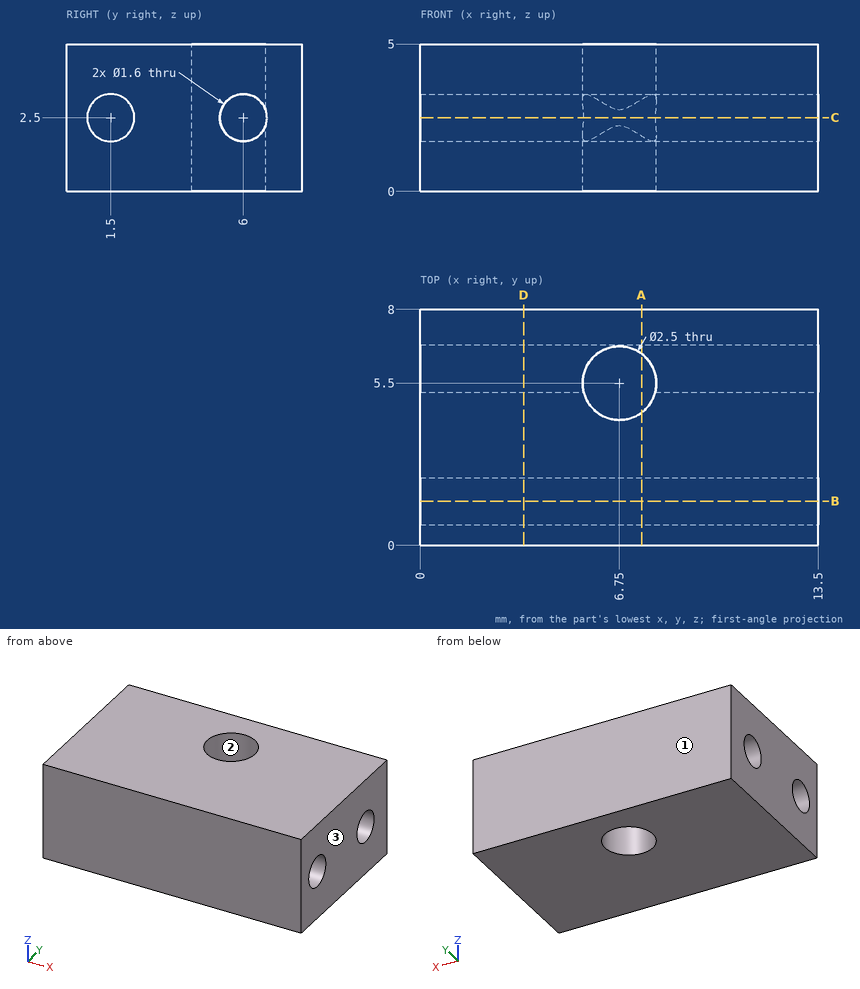
Geometry check sheet. Reference: drawing and pictorial views, mm from the part's lowest x, y, z. Round coordinates to 2 decimals unless told otherwise and drop trailing zeros. Order: outer loops, then holes, each group sorted by start corner. A loop starts at its lowest first (then second) coordinate and runs counter-clockwise, first axis right, second up.
Q1. Cross-section at C-C, the plane z = 2.5. Enter the section's corners in (x, y).
Filled sheet:
outline: (0, 0) - (13.5, 0) - (13.5, 0.7) - (0, 0.7) - close; (0, 2.3) - (13.5, 2.3) - (13.5, 5.2) - (7.96, 5.2) arc R1.25 cw to (5.54, 5.2) - (0, 5.2) - close; (0, 6.8) - (13.5, 6.8) - (13.5, 8) - (0, 8) - close
Q2. Draft check along Y on the marked faces 1, 2 and 3. Enter one of: pulls with the +Y half, pulls with the -Y half, needs draft (parallel to the pull), parting line crosses it, or undercut.
Filled sheet:
face 1: pulls with the +Y half
face 2: undercut
face 3: needs draft
Q3. Cross-section at D-D, the plane x = 3.5. Enter the section's corners in (y, z), plus the area to 3 significant figures.
Filled sheet:
outline: (0, 0) - (8, 0) - (8, 5) - (0, 5) - close; hole circle Ø1.6 at (1.5, 2.5); hole circle Ø1.6 at (6, 2.5)
area: 36.0 mm2
Q4. Cross-section at A-A, the plane x = 7.5. Enter the section's corners in (y, z).
Filled sheet:
outline: (0, 0) - (4.5, 0) - (4.5, 5) - (0, 5) - close; (6.5, 0) - (8, 0) - (8, 5) - (6.5, 5) - (6.5, 3.12) arc R0.8 cw to (6.5, 1.88) - close; hole circle Ø1.6 at (1.5, 2.5)
Q5. Cross-section at B-B, the plane y = 1.5. Enter the section's corners in (x, z), plus the area to 3 significant figures.
Filled sheet:
outline: (0, 0) - (13.5, 0) - (13.5, 1.7) - (0, 1.7) - close; (0, 3.3) - (13.5, 3.3) - (13.5, 5) - (0, 5) - close
area: 45.9 mm2
Q6. Scan lines: L1, parallel to Y at x = 5.5, z = 2.5; L2, parallel to Z at x = 3, y = 6; L3, parallel to X at y = 5.5, z = 1.3. Record each from-to range of solid material in increasing order.
Filled sheet:
L1: y = 0 to 0.7, 2.3 to 5.2, 6.8 to 8
L2: z = 0 to 1.7, 3.3 to 5
L3: x = 0 to 5.5, 8 to 13.5
Q7. Depth check by flat-ended pin: P1, Ø2.5, axis at y = 1.5, z = 2.5, coming from the -X side. Enter the tip coordinate at first touch or a pass-through.
Filled sheet:
P1: stops at x = 0
